from build123d import *

# Parameters (mm, degrees)
SKETCH_1_R      = 6
EXTRUDE_1_DEPTH = 100


with BuildPart() as part:
    # 草图1 → 凸台-拉伸1 (new body)
    with BuildSketch(Plane.XY):
        with BuildLine():
            Line((-28.674392903, 51.362622721), (-47.074392903, 51.362622721))
            ThreePointArc((-47.074392903, 51.362622721), (-48.842159856, 50.630389674), (-49.574392903, 48.862622721))
            Line((-49.574392903, 48.862622721), (-49.574392903, 30.462622721))
            Line((-49.574392903, 30.462622721), (-44.574392903, 30.462622721))
            Line((-44.574392903, 30.462622721), (-44.574392903, 36.862622721))
            Line((-44.574392903, 36.862622721), (-39.458454947, 36.862622721))
            Line((-39.458454947, 36.862622721), (-37.074392903, 34.478560678))
            Line((-37.074392903, 34.478560678), (-37.074392903, 26.362622721))
            Line((-37.074392903, 26.362622721), (-37.074392903, 18.246684764))
            Line((-37.074392903, 18.246684764), (-39.458454947, 15.862622721))
            Line((-39.458454947, 15.862622721), (-44.574392903, 15.862622721))
            Line((-44.574392903, 15.862622721), (-44.574392903, 22.262622721))
            Line((-44.574392903, 22.262622721), (-49.574392903, 22.262622721))
            Line((-49.574392903, 22.262622721), (-49.574392903, 1.362622721))
            Line((-49.574392903, 1.362622721), (-49.574392903, -19.537377279))
            Line((-49.574392903, -19.537377279), (-44.574392903, -19.537377279))
            Line((-44.574392903, -19.537377279), (-44.574392903, -13.137377279))
            Line((-44.574392903, -13.137377279), (-39.458454947, -13.137377279))
            Line((-39.458454947, -13.137377279), (-37.074392903, -15.521439322))
            Line((-37.074392903, -15.521439322), (-37.074392903, -23.637377279))
            Line((-37.074392903, -23.637377279), (-37.074392903, -31.753315236))
            Line((-37.074392903, -31.753315236), (-39.458454947, -34.137377279))
            Line((-39.458454947, -34.137377279), (-44.574392903, -34.137377279))
            Line((-44.574392903, -34.137377279), (-44.574392903, -27.737377279))
            Line((-44.574392903, -27.737377279), (-49.574392903, -27.737377279))
            Line((-49.574392903, -27.737377279), (-49.574392903, -46.137377279))
            ThreePointArc((-49.574392903, -46.137377279), (-48.842159856, -47.905144232), (-47.074392903, -48.637377279))
            Line((-47.074392903, -48.637377279), (-28.674392903, -48.637377279))
            Line((-28.674392903, -48.637377279), (-28.674392903, -43.637377279))
            Line((-28.674392903, -43.637377279), (-35.074392903, -43.637377279))
            Line((-35.074392903, -43.637377279), (-35.074392903, -38.521439322))
            Line((-35.074392903, -38.521439322), (-32.69033086, -36.137377279))
            Line((-32.69033086, -36.137377279), (-24.574392903, -36.137377279))
            Line((-24.574392903, -36.137377279), (-16.458454947, -36.137377279))
            Line((-16.458454947, -36.137377279), (-14.074392903, -38.521439322))
            Line((-14.074392903, -38.521439322), (-14.074392903, -43.637377279))
            Line((-14.074392903, -43.637377279), (-20.474392903, -43.637377279))
            Line((-20.474392903, -43.637377279), (-20.474392903, -48.637377279))
            Line((-20.474392903, -48.637377279), (0.425607097, -48.637377279))
            Line((0.425607097, -48.637377279), (21.325607097, -48.637377279))
            Line((21.325607097, -48.637377279), (21.325607097, -43.637377279))
            Line((21.325607097, -43.637377279), (14.925607097, -43.637377279))
            Line((14.925607097, -43.637377279), (14.925607097, -38.521439322))
            Line((14.925607097, -38.521439322), (17.30966914, -36.137377279))
            Line((17.30966914, -36.137377279), (25.425607097, -36.137377279))
            Line((25.425607097, -36.137377279), (33.541545053, -36.137377279))
            Line((33.541545053, -36.137377279), (35.925607097, -38.521439322))
            Line((35.925607097, -38.521439322), (35.925607097, -43.637377279))
            Line((35.925607097, -43.637377279), (29.525607097, -43.637377279))
            Line((29.525607097, -43.637377279), (29.525607097, -48.637377279))
            Line((29.525607097, -48.637377279), (47.925607097, -48.637377279))
            ThreePointArc((47.925607097, -48.637377279), (49.69337405, -47.905144232), (50.425607097, -46.137377279))
            Line((50.425607097, -46.137377279), (50.425607097, -27.737377279))
            Line((50.425607097, -27.737377279), (45.425607097, -27.737377279))
            Line((45.425607097, -27.737377279), (45.425607097, -34.137377279))
            Line((45.425607097, -34.137377279), (40.30966914, -34.137377279))
            Line((40.30966914, -34.137377279), (37.925607097, -31.753315236))
            Line((37.925607097, -31.753315236), (37.925607097, -23.637377279))
            Line((37.925607097, -23.637377279), (37.925607097, -15.521439322))
            Line((37.925607097, -15.521439322), (40.30966914, -13.137377279))
            Line((40.30966914, -13.137377279), (45.425607097, -13.137377279))
            Line((45.425607097, -13.137377279), (45.425607097, -19.537377279))
            Line((45.425607097, -19.537377279), (50.425607097, -19.537377279))
            Line((50.425607097, -19.537377279), (50.425607097, 1.362622721))
            Line((50.425607097, 1.362622721), (50.425607097, 22.262622721))
            Line((50.425607097, 22.262622721), (45.425607097, 22.262622721))
            Line((45.425607097, 22.262622721), (45.425607097, 15.862622721))
            Line((45.425607097, 15.862622721), (40.30966914, 15.862622721))
            Line((40.30966914, 15.862622721), (37.925607097, 18.246684764))
            Line((37.925607097, 18.246684764), (37.925607097, 26.362622721))
            Line((37.925607097, 26.362622721), (37.925607097, 34.478560678))
            Line((37.925607097, 34.478560678), (40.30966914, 36.862622721))
            Line((40.30966914, 36.862622721), (45.425607097, 36.862622721))
            Line((45.425607097, 36.862622721), (45.425607097, 30.462622721))
            Line((45.425607097, 30.462622721), (50.425607097, 30.462622721))
            Line((50.425607097, 30.462622721), (50.425607097, 48.862622721))
            ThreePointArc((50.425607097, 48.862622721), (49.69337405, 50.630389674), (47.925607097, 51.362622721))
            Line((47.925607097, 51.362622721), (29.525607097, 51.362622721))
            Line((29.525607097, 51.362622721), (29.525607097, 46.362622721))
            Line((29.525607097, 46.362622721), (35.925607097, 46.362622721))
            Line((35.925607097, 46.362622721), (35.925607097, 41.246684764))
            Line((35.925607097, 41.246684764), (33.541545053, 38.862622721))
            Line((33.541545053, 38.862622721), (25.425607097, 38.862622721))
            Line((25.425607097, 38.862622721), (17.30966914, 38.862622721))
            Line((17.30966914, 38.862622721), (14.925607097, 41.246684764))
            Line((14.925607097, 41.246684764), (14.925607097, 46.362622721))
            Line((14.925607097, 46.362622721), (21.325607097, 46.362622721))
            Line((21.325607097, 46.362622721), (21.325607097, 51.362622721))
            Line((21.325607097, 51.362622721), (0.425607097, 51.362622721))
            Line((0.425607097, 51.362622721), (-20.474392903, 51.362622721))
            Line((-20.474392903, 51.362622721), (-20.474392903, 46.362622721))
            Line((-20.474392903, 46.362622721), (-14.074392903, 46.362622721))
            Line((-14.074392903, 46.362622721), (-14.074392903, 41.246684764))
            Line((-14.074392903, 41.246684764), (-16.458454947, 38.862622721))
            Line((-16.458454947, 38.862622721), (-24.574392903, 38.862622721))
            Line((-24.574392903, 38.862622721), (-32.69033086, 38.862622721))
            Line((-32.69033086, 38.862622721), (-35.074392903, 41.246684764))
            Line((-35.074392903, 41.246684764), (-35.074392903, 46.362622721))
            Line((-35.074392903, 46.362622721), (-28.674392903, 46.362622721))
            Line((-28.674392903, 46.362622721), (-28.674392903, 51.362622721))
        make_face()
        with Locations((-24.574392903, 26.362622721)):
            Circle(SKETCH_1_R, mode=Mode.SUBTRACT)
        with Locations((25.425607097, 26.362622721)):
            Circle(SKETCH_1_R, mode=Mode.SUBTRACT)
        with Locations((-24.574392903, -23.637377279)):
            Circle(SKETCH_1_R, mode=Mode.SUBTRACT)
        with Locations((25.425607097, -23.637377279)):
            Circle(SKETCH_1_R, mode=Mode.SUBTRACT)
        with BuildLine():
            Line((-35.826372672, 39.735922833), (-39.541550191, 43.451100352))
            ThreePointArc((-39.541550191, 43.451100352), (-43.784190878, 45.572420696), (-41.662870534, 41.329780008))
            Line((-41.662870534, 41.329780008), (-37.947693016, 37.61460249))
            Line((-37.947693016, 37.61460249), (-35.826372672, 39.735922833))
        make_face(mode=Mode.SUBTRACT)
        Polygon((-8.074392903, 45.362622721), (-8.074392903, 38.76140339), (-12.574392903, 34.26140339), (-12.574392903, 23.362622721), (-21.574392903, 14.362622721), (-32.473173572, 14.362622721), (-36.973173572, 9.862622721), (-43.574392903, 9.862622721), (-43.574392903, 1.362622721), (-43.574392903, -7.137377279), (-36.973173572, -7.137377279), (-32.473173572, -11.637377279), (-21.574392903, -11.637377279), (-12.574392903, -20.637377279), (-12.574392903, -31.536157948), (-8.074392903, -36.036157948), (-8.074392903, -42.637377279), (0.425607097, -42.637377279), (8.925607097, -42.637377279), (8.925607097, -36.036157948), (13.425607097, -31.536157948), (13.425607097, -20.637377279), (22.425607097, -11.637377279), (33.324387766, -11.637377279), (37.824387766, -7.137377279), (44.425607097, -7.137377279), (44.425607097, 1.362622721), (44.425607097, 9.862622721), (37.824387766, 9.862622721), (33.324387766, 14.362622721), (22.425607097, 14.362622721), (13.425607097, 23.362622721), (13.425607097, 34.26140339), (8.925607097, 38.76140339), (8.925607097, 45.362622721), (0.425607097, 45.362622721), align=None, mode=Mode.SUBTRACT)
        with BuildLine():
            Line((36.677586865, 39.735922833), (40.392764384, 43.451100352))
            ThreePointArc((40.392764384, 43.451100352), (44.635405071, 45.572420696), (42.514084728, 41.329780008))
            Line((42.514084728, 41.329780008), (38.798907209, 37.61460249))
            Line((38.798907209, 37.61460249), (36.677586865, 39.735922833))
        make_face(mode=Mode.SUBTRACT)
        with BuildLine():
            Line((-35.826372672, -37.010677391), (-39.541550191, -40.72585491))
            ThreePointArc((-39.541550191, -40.72585491), (-43.784190878, -42.847175254), (-41.662870534, -38.604534567))
            Line((-41.662870534, -38.604534567), (-37.947693016, -34.889357048))
            Line((-37.947693016, -34.889357048), (-35.826372672, -37.010677391))
        make_face(mode=Mode.SUBTRACT)
        with BuildLine():
            Line((36.677586865, -37.010677391), (40.392764384, -40.72585491))
            ThreePointArc((40.392764384, -40.72585491), (44.635405071, -42.847175254), (42.514084728, -38.604534567))
            Line((42.514084728, -38.604534567), (38.798907209, -34.889357048))
            Line((38.798907209, -34.889357048), (36.677586865, -37.010677391))
        make_face(mode=Mode.SUBTRACT)
    extrude(amount=EXTRUDE_1_DEPTH)


solid = part.part
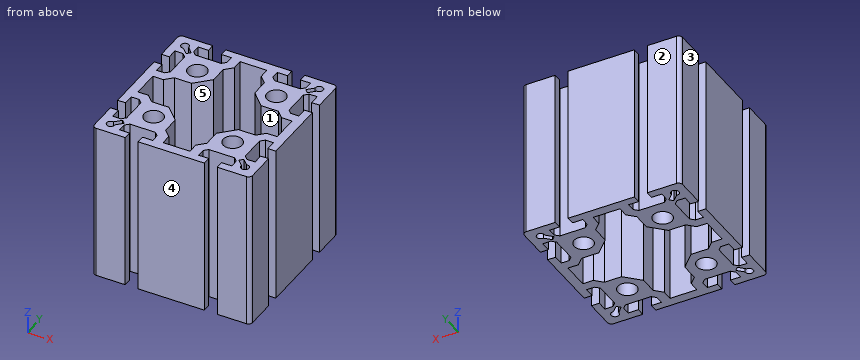
Could you check a few things on this model? Use its own coordinates, in mm. Face numbers are marked on the shaded views. A direction names the side the tool comes from. Give positions to 0.01 mm unless a question says otherwise; leave off trailing zeros. Order: outer loops, then holes, each group sorted by start corner. A loop starts at its lowest first (then second) coordinate and runs counter-clockwise, first axis right, second up. Notation, with made-up numbers: (42, 8.5) - (80, 8.5) arc R27 ccw to (80, 24.5) - close; hole circle Ø4 at (69.5, -32). An arc over 180 degrees is marked (long way). One line per item, written item: value. Start each with the question number.
1. For the marked faces 1 and 2, which set-ups out of +Z, -Z, +X, -X, +Y, -Y let a thin tool reach every point of the face, with its end or its side?
2. Thinking about a two-plate mould opening in Y: for the marked faces 3, 4 and 5, which applies, +Y half, -Y half, draft (parallel to the pull), parting line (faces both ways), or undercut?
3. Imagine slicing it at A-A on y = 8. List the corners of the cut face in (x, z) for me.
4. Imagine slicing it at C-C on x = -25. List the corners of the cut face in (y, z) for me.
5. If I drill on probe 1 along Y at (x, z) = (-25, 66.5); probe 2 along Y at (x, z) = (33, 26); probe 3 along Y at (x, z) = (-45, 8), over which ranges is the centre line in solid material (lowest first)?
6. Imagine slicing it at D-D on x = 24.5. List the corners of the cut face in (y, z) for me, plus the area to 3 significant figures.
7. Imagine slicing it at B-B on x = -2. List the corners of the cut face in (y, z) for me, plus the area to 3 significant figures.
Values:
1. face 1: +Z, -Z
1. face 2: +Z, -Z, +X, -X, +Y
2. face 3: draft
2. face 4: -Y half
2. face 5: undercut
3. outline: (-49.57, 0) - (-43.57, 0) - (-43.57, 100) - (-49.57, 100) - close; (44.43, 0) - (50.43, 0) - (50.43, 100) - (44.43, 100) - close
4. outline: (-36.14, 0) - (-29.62, 0) - (-29.62, 100) - (-36.14, 100) - close; (-17.65, 0) - (-11.64, 0) - (-11.64, 100) - (-17.65, 100) - close; (14.36, 0) - (20.38, 0) - (20.38, 100) - (14.36, 100) - close; (32.35, 0) - (38.86, 0) - (38.86, 100) - (32.35, 100) - close
5. probe 1: -36.14 to -29.62, -17.65 to -11.64, 14.36 to 20.38, 32.35 to 38.86
5. probe 2: -48.64 to -43.64, -36.14 to -11.64, 14.36 to 38.86, 46.36 to 51.36
5. probe 3: -48.64 to -27.74, -19.54 to 22.26, 30.46 to 51.36
6. outline: (-36.14, 0) - (-29.57, 0) - (-29.57, 100) - (-36.14, 100) - close; (-17.71, 0) - (-11.64, 0) - (-11.64, 100) - (-17.71, 100) - close; (14.36, 0) - (20.43, 0) - (20.43, 100) - (14.36, 100) - close; (32.29, 0) - (38.86, 0) - (38.86, 100) - (32.29, 100) - close
6. area: 2,530 mm²
7. outline: (-48.64, 0) - (-42.64, 0) - (-42.64, 100) - (-48.64, 100) - close; (45.36, 0) - (51.36, 0) - (51.36, 100) - (45.36, 100) - close
7. area: 1,200 mm²
